from build123d import *

# Parameters (mm, degrees)
BOSS_EXTRUDE2_DEPTH           = 18
BOSS_EXTRUDE2_DEPTH_BACK      = 6
BOSS_EXTRUDE3_DEPTH           = 18
BOSS_EXTRUDE3_DEPTH_BACK      = 6
LOAD_BAR_ARM_SLOTS_DEPTH      = 30
LOAD_BAR_ARM_SLOTS_DEPTH_BACK = 30
F_10KG_START                  = 1.4
F_10KG_TAL_BAR_SLOT_DEPTH     = 16.6
HX711_CHIP_HOLSTER_DEPTH      = 18
HX711_CHIP_HOLSTER_DEPTH_BACK = 4.6
SKETCH6_R                     = 1.8
SCREW_HOLE_DEPTH              = 18
CHAMFER3_SIZE                 = 0.4
CHAMFER8_SIZE                 = 1
CUT_EXTRUDE6_DEPTH            = 7
CUT_EXTRUDE6_DEPTH_BACK       = 7


with BuildPart() as part:
    # Sketch1 → Boss-Extrude2 (new, two sides: drawn at the far end of the back side and taken through both)
    with BuildSketch(Plane(origin=(0, 0, 0), x_dir=(1, 0, 0), z_dir=(0, 1, 0)).offset(-BOSS_EXTRUDE2_DEPTH_BACK)):
        with BuildLine():
            Line((-41.5, 14), (41.5, 14))
            ThreePointArc((41.5, 14), (42.207106781, 13.707106781), (42.5, 13))
            Line((42.5, 13), (42.5, -13))
            ThreePointArc((42.5, -13), (42.207106781, -13.707106781), (41.5, -14))
            Line((41.5, -14), (-41.5, -14))
            ThreePointArc((-41.5, -14), (-42.207106781, -13.707106781), (-42.5, -13))
            Line((-42.5, -13), (-42.5, 13))
            ThreePointArc((-42.5, 13), (-42.207106781, 13.707106781), (-41.5, 14))
        make_face()
    extrude(amount=BOSS_EXTRUDE2_DEPTH + BOSS_EXTRUDE2_DEPTH_BACK)

    # Sketch4 → Boss-Extrude3 (add, two sides: drawn at the far end of the back side and taken through both)
    with BuildSketch(Plane(origin=(0, 0, 0), x_dir=(1, 0, 0), z_dir=(0, 1, 0)).offset(-BOSS_EXTRUDE3_DEPTH_BACK)):
        Polygon((-12.5, 23), (12.5, 23), (22.5, 14), (22.5, -14), (12.5, -23), (-12.5, -23), (-22.5, -14), (-22.5, 14), align=None)
    extrude(amount=BOSS_EXTRUDE3_DEPTH + BOSS_EXTRUDE3_DEPTH_BACK)

    # Sketch2 → load bar arm slots (cut, two sides: drawn at the far end of the back side and taken through both)
    with BuildSketch(Plane.XY.offset(-LOAD_BAR_ARM_SLOTS_DEPTH_BACK)):
        with BuildLine():
            Line((-3.5, 19), (3.5, 19))
            ThreePointArc((3.5, 19), (4.207106781, 18.707106781), (4.5, 18))
            Line((4.5, 18), (4.5, 1))
            ThreePointArc((4.5, 1), (4.207106781, 0.292893219), (3.5, 0))
            Line((3.5, 0), (-3.5, 0))
            ThreePointArc((-3.5, 0), (-4.207106781, 0.292893219), (-4.5, 1))
            Line((-4.5, 1), (-4.5, 18))
            ThreePointArc((-4.5, 18), (-4.207106781, 18.707106781), (-3.5, 19))
        make_face()
    extrude(amount=LOAD_BAR_ARM_SLOTS_DEPTH + LOAD_BAR_ARM_SLOTS_DEPTH_BACK, mode=Mode.SUBTRACT)

    # Sketch5 → 10kg TAL bar slot (cut)
    with BuildSketch(Plane(origin=(0, 0, 0), x_dir=(1, 0, 0), z_dir=(0, 1, 0)).offset(F_10KG_START)):
        with BuildLine():
            Line((-40.5, 8), (-40.5, -11.01888353))
            ThreePointArc((-40.5, -11.01888353), (-40.212637639, -11.712637639), (-39.51888353, -12))
            Line((-39.51888353, -12), (13.495093721, -12))
            Line((13.495093721, -12), (13.495093721, -8))
            Line((13.495093721, -8), (40.495093721, -8))
            Line((40.495093721, -8), (40.495093721, 10.991511742))
            ThreePointArc((40.495093721, 10.991511742), (40.196297826, 11.708039924), (39.4769572, 12))
            Line((39.4769572, 12), (-13.5, 12))
            Line((-13.5, 12), (-13.5, 8))
            Line((-13.5, 8), (-40.5, 8))
        make_face()
    extrude(amount=F_10KG_TAL_BAR_SLOT_DEPTH, mode=Mode.SUBTRACT)

    # Sketch3 → hx711 chip holster (cut, two sides: drawn at the far end of the back side and taken through both)
    with BuildSketch(Plane(origin=(0, 0, 0), x_dir=(1, 0, 0), z_dir=(0, 1, 0)).offset(-HX711_CHIP_HOLSTER_DEPTH_BACK)):
        Polygon((-2.622290437, 20.931402076), (-19.822831867, 7.214938445), (2.622290437, -20.931402076), (19.822831867, -7.214938445), align=None)
    extrude(amount=HX711_CHIP_HOLSTER_DEPTH + HX711_CHIP_HOLSTER_DEPTH_BACK, mode=Mode.SUBTRACT)

    # Sketch6 → screw hole (cut)
    with BuildSketch(Plane(origin=(0, 0, 0), x_dir=(1, 0, 0), z_dir=(0, 1, 0))):
        with Locations(Location((-10, -17, 0), (0, 0, 270))):
            Circle(SKETCH6_R)
        with Locations(Location((10, 17, 0), (0, 0, 270))):
            Circle(SKETCH6_R)
    extrude(amount=SCREW_HOLE_DEPTH, mode=Mode.SUBTRACT)

    # Chamfer3
    chamfer3_edges = [part.edges().sort_by_distance(p)[0] for p in [
        (-10, 18, 15.2),
        (10, 18, -18.8),
        (42.207106781, 18, -13.707106781),
        (32, 18, -14),
        (-42.207106781, 18, -13.707106781),
        (-42.5, 18, 0),
        (-42.207106781, 18, 13.707106781),
        (-32, 18, 14),
        (42.207106781, 18, 13.707106781),
        (42.5, 18, 0),
        (-32, 18, -14),
        (32, 18, 14),
        (-17.5, 18, 18.5),
        (-8.5, 18, 23),
        (17.5, 18, 18.5),
        (17.5, 18, -18.5),
        (8.5, 18, -23),
        (-17.5, 18, -18.5),
        (8.5, 18, 23),
        (4.5, 9.5, 23),
        (4.207106781, 0.292893219, 23),
        (0, 0, 23),
        (-4.207106781, 0.292893219, 23),
        (-4.5, 9.5, 23),
        (-8.5, 18, -23),
        (4.5, 9.5, -23),
        (-4.5, 9.5, -23),
        (-4.207106781, 0.292893219, -23),
        (0, 0, -23),
        (4.207106781, 0.292893219, -23),
    ]]
    chamfer(chamfer3_edges, length=CHAMFER3_SIZE)

    # Chamfer8
    chamfer8_edges = [part.edges().sort_by_distance(p)[0] for p in [
        (-42.207106781, -6, -13.707106781),
        (-42.5, -6, 0),
        (-42.207106781, -6, 13.707106781),
        (-32, -6, 14),
        (42.207106781, -6, 13.707106781),
        (42.5, -6, 0),
        (32, -6, 14),
        (-32, -6, -14),
        (-17.5, -6, -18.5),
        (0, -6, -23),
        (17.5, -6, -18.5),
        (42.207106781, -6, -13.707106781),
        (17.5, -6, 18.5),
        (0, -6, 23),
        (-17.5, -6, 18.5),
        (32, -6, -14),
    ]]
    chamfer(chamfer8_edges, length=CHAMFER8_SIZE - 0.0001)  # a hair under: the kernel refuses the full size

    # Sketch10 → Cut-Extrude6 (cut, two sides: drawn at the far end of the back side and taken through both)
    with BuildSketch(Plane(origin=(0, 0, 0), x_dir=(1, 0, 0), z_dir=(0, 1, 0)).offset(-CUT_EXTRUDE6_DEPTH_BACK)):
        with BuildLine():
            Line((-38, -5), (-38, 5))
            ThreePointArc((-38, 5), (-36, 7), (-34, 5))
            Line((-34, 5), (-34, -5))
            ThreePointArc((-34, -5), (-36, -7), (-38, -5))
        make_face()
        with BuildLine():
            Line((-31.5, -5), (-31.5, 5))
            ThreePointArc((-31.5, 5), (-29.5, 7), (-27.5, 5))
            Line((-27.5, 5), (-27.5, -5))
            ThreePointArc((-27.5, -5), (-29.5, -7), (-31.5, -5))
        make_face()
        with BuildLine():
            Line((-25, -5), (-25, 5))
            ThreePointArc((-25, 5), (-23, 7), (-21, 5))
            Line((-21, 5), (-21, -5))
            ThreePointArc((-21, -5), (-23, -7), (-25, -5))
        make_face()
        with BuildLine():
            Line((21, -5), (21, 5))
            ThreePointArc((21, 5), (23, 7), (25, 5))
            Line((25, 5), (25, -5))
            ThreePointArc((25, -5), (23, -7), (21, -5))
        make_face()
        with BuildLine():
            Line((27.5, -5), (27.5, 5))
            ThreePointArc((27.5, 5), (29.5, 7), (31.5, 5))
            Line((31.5, 5), (31.5, -5))
            ThreePointArc((31.5, -5), (29.5, -7), (27.5, -5))
        make_face()
        with BuildLine():
            Line((34, -5), (34, 5))
            ThreePointArc((34, 5), (36, 7), (38, 5))
            Line((38, 5), (38, -5))
            ThreePointArc((38, -5), (36, -7), (34, -5))
        make_face()
    extrude(amount=CUT_EXTRUDE6_DEPTH + CUT_EXTRUDE6_DEPTH_BACK, mode=Mode.SUBTRACT)


solid = part.part
Could you check a few things on this model? Use its own coordinates, in mm. A direction names the side the tool comes from. Coordinates: 2 decimals unless noted, no trailing zeros. Loops run counter-clockwise (first coordinate to the right, second up) from the corner with the lowest first, then second, coordinate; pieces in that order, holes last. Notation, with made-up numbers: (-36, 31.5) -> (-16, 31.5) arc R19 ccw to (-16, 40.5) -> close; hole circle Ø1 at (43.25, 59). An arc over 180 degrees is marked (long way). Answer in a Markdown table with one row per item.
(1) Thinking about a two-plate mould opening in X: for faces 6 (the face through (-17.354, 17.797, 18.366)), 7 (the face through (-8.76, -1.64, 6.66)), 8 (the face through (6, 6, 23)), 9 (the face through (17.2, -5.5, -18.1)), which applies, released by +X, released by -X, zero draft, split by the parting line, or undercut?
Results found:
| item | result |
|---|---|
| face 6 | released by -X |
| face 7 | undercut |
| face 8 | zero draft |
| face 9 | released by +X |
(2) Imagine slicing it at A-A (x = -36). List the corners of the cut face in (y, z) for me, plus the area to 3 significant figures.
Results found:
| item | result |
|---|---|
| outline | (-6, -13) -> (-5, -14) -> (17.6, -14) -> (18, -13.6) -> (18, -8) -> (1.4, -8) -> (1.4, -7) -> (-6, -7) -> close; (-6, 7) -> (1.4, 7) -> (1.4, 12) -> (18, 12) -> (18, 13.6) -> (17.6, 14) -> (-5, 14) -> (-6, 13) -> close |
| area | 235 mm^2 |
(3) Will these pins go through, and if not, where does the flat tip stop? pin 1 Ø6 at (x, y) = (-27, 8) entering from -Z; pin 2 Ø1.5 at (y, z) = (1.5, 16.5) entering from +X; pin 3 Ø1 at (x, z) = (-27.5, -2) entering from +Y.
Results found:
| item | result |
|---|---|
| pin 1 | stops at z = -14 |
| pin 2 | stops at x = 20.56 |
| pin 3 | stops at y = 1.4 |
(4) For faces 1 (the face through (-17.2, -5.5, 18.1)), 2 (the face through (34, -2, 0)), 3 (the face through (-20.4, 18, -8.5)), 4 (the face through (4.5, 10, 21)), 5 (the face through (30, 10, 8)), which set-ups out of +Z, -Z, +X, -X, +Y, -Y let a thin tool reach every point of the face, with its end or its side?
Results found:
| item | result |
|---|---|
| face 1 | +Z, -X, -Y |
| face 2 | +Y, -Y |
| face 3 | +Z, -Z, +X, -X, +Y |
| face 4 | +Z, -Z, +Y |
| face 5 | +Y |
(5) Imagine slicing it at B-B (y = 15). Give the number of separate pieces and of enclosed holes in the cut face, plus the area to 3 significant figures.
Results found:
| item | result |
|---|---|
| separate pieces | 2 |
| enclosed holes | 2 |
| area | 971 mm^2 |
(6) Imagine slicing it at D-D (x = -1.5). List the corners of the cut face in (y, z) for me.
Results found:
| item | result |
|---|---|
| outline | (-6, -22) -> (-5, -23) -> (-0.4, -23) -> (0, -22.6) -> (0, -19.52) -> (-4.6, -19.52) -> (-4.6, 15.76) -> (0, 15.76) -> (0, 22.6) -> (-0.4, 23) -> (-5, 23) -> (-6, 22) -> close |
(7) If I drill on probe 1 along X at (y, z) = (2, -16); probe 2 along X at (y, z) = (12, 18.5); probe 3 along Z at (x, y) = (-30, 10.75), over which ranges is the centre line in solid material (lowest first)?
Results found:
| item | result |
|---|---|
| probe 1 | x = -20.28 to -8.81, 4.5 to 8.5, 11.5 to 20.28 |
| probe 2 | x = -17.5 to -10.99, -9.01 to -4.5, 5.67 to 17.5 |
| probe 3 | z = -14 to -8, 12 to 14 |
